Solid Edge part; units mm, degrees
sketch "Sketch1" plane through (0, 0, 0) normal (0, 0, 1) x (1, 0, 0)
  circle A0 centre (0, 0) radius 22.098
extrude "Protrusion1" add sketch "Sketch1" along normal blind 15.9258
sketch "Sketch2" plane through (0, 0, 0) normal (0, 0, -1) x (1, 0, 0)
  circle A0 centre (0, 0) radius 12.7
extrude "Protrusion2" add sketch "Sketch2" along normal blind 88.9
sketch "Sketch3" plane through (0, 0, -88.9) normal (0, 0, -1) x (1, 0, 0)
  circle A0 centre (0, 0) radius 12.6997
extrude "Cutout1" cut sketch "Sketch3" against normal blind 57.15 flip side to cut
chamfer "Chamfer_1" distance 1.905 angle 45 1 edges at (-12.6997, 0, -88.9)
sketch "Sketch4" plane through (0, 0, 15.9258) normal (0, 0, 1) x (1, 0, 0)
  line L0 (-11.1991, 19.05) -> (11.1991, 19.05)
extrude "Cutout2" cut sketch "Sketch4" against normal up to next material side at (0, 19.1, 15.9258)
pattern_circular "Pattern1" count 6 over 360 about axis through (0, 0, 15.9258) along (0, 0, 1) of "Cutout2"
properties part number "24107015"
Can you work these out from the model? Positions are in its coordinate system, mm. A direction names the side the tool comes from. Coordinates: 2 decimals unless noted, no trailing zeros. Write each loop counter-clockwise with the first axis right and the second up, starting at its lowest first coordinate (ties: lowest second). Pieces come first, ordered by that corner, then holes. Notation, with made-up numbers: (86.5, 4.5) -> (98.5, 4.5) arc R11 cw to (98.5, 18.5) -> close; hole circle Ø7 at (63.5, 48). An arc over 180 degrees is marked (long way). Answer as CSV lines item,"result".
1) If I drill on line 1 (Z direction, x = 4.5, y = 14.5); line 2 (X direction, y = -0.5, z = -44); line 3 (X direction, y = 6.5, z = -48), over which ranges is the centre line in solid material (lowest first)? Write a range as from..to.
Check result:
line 1,"0..15.93"
line 2,"-12.69..12.69"
line 3,"-10.91..10.91"
2) On a 3-axis mill with a long thin cutter (end or side, diameter ignored), from which of +Z, -Z, +X, -X, +Y, -Y can I reach the whole of each face in a straight line? I mean faces 1 (the cylindrical face through (-2.75, -12.4, -15.65)), 2 (the flat face through (16.575, -9.392, 8.074)). Say none if no direction works.
Check result:
face 1,"-Z"
face 2,"+Z, -Z, +X, -Y"
3) Will these pins go through, and if not, where does the flat tip stop? P1, Ø6, axis at y = -3, z = -14.5, coming from the -X side; P2, Ø10, axis at y = -6, z = -76, coming from the +X side; P3, Ø8, axis at x = -10.5, z = -39.5, coming from the +Y side.
Check result:
P1,"x = -12.7"
P2,"x = 12.66"
P3,"y = 10.91"
4) If we section it at B-B on z = -15.5: Please give me the cut outline in (x, y).
Check result:
outline,"circle Ø25.4 at (0, 0)"
5) If we section it at C-C on y = 15.5: Please give me the cut outline in (x, z), then the cut area to 3 significant figures.
Check result:
outline,"(-13.05, 0) -> (13.05, 0) -> (13.05, 15.93) -> (-13.05, 15.93) -> close"
area,"416 mm²"
